Could you check a few things on this model? Use its own coordinates, in mm. Face numbers are marked on the shaded views. A direction names the side the tool comes from. Coordinates: 2 decimals unless noted, no trailing zeros. Order: outer loops, then holes, each group sorted by start corner. A loop starts at its lowest first (then second) coordinate and runs counter-clockwise, first axis right, second up. Notation, with made-up numbers: (-13, 49) - (13, 49) arc R22 cw to (13, 63) - close; hole circle Ø1 at (-26, 11.25). An arc over 180 degrees is marked (long way). One line per item, written item: value.
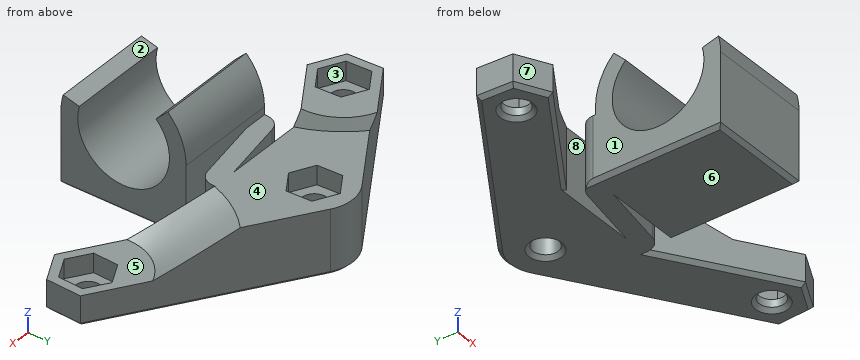
from build123d import *

# Parameters (mm, degrees)
BOSS_EXTRUDE1_DEPTH = 13.5
CUT_EXTRUDE1_DEPTH  = 19.454335534
SKETCH14_R          = 1.65
BOSS_EXTRUDE3_DEPTH = 8.5
CUT_EXTRUDE7_DEPTH  = 43.153930156
FILLET2_R           = 2
CUT_EXTRUDE9_DEPTH  = 4.5
CHAMFER2_SIZE       = 12
CHAMFER2_SIZE_2     = 6
CHAMFER3_SIZE       = 6
CHAMFER3_SIZE_2     = 12
CUT_EXTRUDE11_DEPTH = 2.5
CUT_EXTRUDE12_DEPTH = 2.5
CHAMFER4_SIZE       = 0.5
CHAMFER8_SIZE       = 0.5


with BuildPart() as part:
    # Sketch1 → Boss-Extrude1 (new body)
    with BuildSketch(Plane.ZY):
        with BuildLine():
            Line((-9.5, 8.25), (-9.5, -8.25))
            Line((-9.5, -8.25), (0, -8.25))
            ThreePointArc((0, -8.25), (8.25, 0), (0, 8.25))
            Line((0, 8.25), (-9.5, 8.25))
        make_face()
    extrude(amount=BOSS_EXTRUDE1_DEPTH)

    # Sketch7 → Cut-Extrude1 (cut, through all)
    with BuildSketch(Plane.ZY.offset(13.5)):
        with BuildLine():
            Line((13.481907846, 13.481907846), (4.277996026, 4.277996026))
            ThreePointArc((4.277996026, 4.277996026), (-5.843851249, 1.565855223), (1.565855223, -5.843851249))
            Line((1.565855223, -5.843851249), (4.934720763, -18.416628609))
            Line((4.934720763, -18.416628609), (13.481907846, 13.481907846))
        make_face()
    extrude(amount=-CUT_EXTRUDE1_DEPTH, mode=Mode.SUBTRACT)

    # Sketch14 → Boss-Extrude3 (add)
    with BuildSketch(Plane(origin=(0, 0, -9.5), x_dir=(-1, 0, 0), z_dir=(0, 0, -1))):
        with BuildLine():
            Line((4.039848555, 24.201794753), (-19.358847021, 9.109670469))
            Line((-19.358847021, 9.109670469), (-19.131451731, 4.496469334))
            Line((-19.131451731, 4.496469334), (-15.022604709, 2.386798865))
            Line((-15.022604709, 2.386798865), (0, 12.07635684))
            Line((0, 12.07635684), (0, 8.25))
            Line((0, 8.25), (13.5, 8.25))
            Line((13.5, 8.25), (13.5, 12.07635684))
            Line((13.5, 12.07635684), (28.522604709, 2.386798865))
            Line((28.522604709, 2.386798865), (32.631451731, 4.496469334))
            Line((32.631451731, 4.496469334), (32.858847021, 9.109670469))
            Line((32.858847021, 9.109670469), (9.460151445, 24.201794753))
            ThreePointArc((9.460151445, 24.201794753), (6.75, 25), (4.039848555, 24.201794753))
        make_face()
        with Locations((6.75, 20)):
            Circle(SKETCH14_R, mode=Mode.SUBTRACT)
        with Locations((-15.25, 7)):
            Circle(SKETCH14_R, mode=Mode.SUBTRACT)
        with Locations(Location((28.75, 7, 0), (0, 0, 180))):
            Circle(SKETCH14_R, mode=Mode.SUBTRACT)
    extrude(amount=-BOSS_EXTRUDE3_DEPTH)

    # Sketch15 → Cut-Extrude7 (cut, through all)
    with BuildSketch(Plane.XY.offset(-1)):
        Polygon((0, 8.25), (-10.401710887, 8.25), (0, 10.084102275), align=None)
        Polygon((-13.5, 10.242254565), (-13.5, 12.07635684), (-3.098289113, 12.07635684), align=None)
    extrude(amount=-CUT_EXTRUDE7_DEPTH, mode=Mode.SUBTRACT)

    # Fillet2
    fillet2_edges = [part.edges().sort_by_distance(p)[0] for p in [
        (0, 10.084102275, -5.25),
        (-13.5, 10.242254565, -5.25),
    ]]
    fillet(fillet2_edges, radius=FILLET2_R)

    # Sketch17 → Cut-Extrude9 (cut)
    with BuildSketch(Plane.XY.offset(-1)):
        with BuildLine():
            Line((19.131451731, 4.496469334), (19.358847021, 9.109670469))
            Line((19.358847021, 9.109670469), (17.418121156, 10.361435802))
            ThreePointArc((17.418121156, 10.361435802), (11.888564198, 9.168121156), (13.081878844, 3.638564198))
            Line((13.081878844, 3.638564198), (15.022604709, 2.386798865))
            Line((15.022604709, 2.386798865), (19.131451731, 4.496469334))
        make_face()
        with BuildLine():
            Line((-32.631451731, 4.496469334), (-28.522604709, 2.386798865))
            Line((-28.522604709, 2.386798865), (-26.581878844, 3.638564198))
            ThreePointArc((-26.581878844, 3.638564198), (-25.388564198, 9.168121156), (-30.918121156, 10.361435802))
            Line((-30.918121156, 10.361435802), (-32.858847021, 9.109670469))
            Line((-32.858847021, 9.109670469), (-32.631451731, 4.496469334))
        make_face()
    extrude(amount=-CUT_EXTRUDE9_DEPTH, mode=Mode.SUBTRACT)

    # Chamfer2
    # the kernel refuses this chamfer: 12, 6 mm, written as the material it takes off along each edge
    with BuildSketch(Plane(origin=(-28.75, 7, -1), x_dir=(-0.8386519680093931, -0.5446676753342096, 0), z_dir=(-0.5446676753342096, 0.8386519680093931, 0))) as chamfer2_piece_1_section:
        Polygon((4 + CHAMFER2_SIZE, 0), (4, -CHAMFER2_SIZE_2), (4, 0), align=None)
    chamfer2_piece_1 = revolve(axis=Axis((-28.75, 7, -1), (0, 0, 1)), revolution_arc=359.64, mode=Mode.PRIVATE)
    chamfer2_piece_1 = split(chamfer2_piece_1, bisect_by=Plane(origin=(-26.581878844, 3.638564198, -1), z_dir=(-0.5420302889814643, 0.8403589505840171, 0)), keep=Keep.TOP, mode=Mode.PRIVATE)
    chamfer2_piece_1 = split(chamfer2_piece_1, bisect_by=Plane(origin=(-28.75, 7, -5.5), z_dir=(0, 0, 1)), keep=Keep.TOP, mode=Mode.PRIVATE)
    add(chamfer2_piece_1, mode=Mode.SUBTRACT)

    # Chamfer3
    # the kernel refuses this chamfer: 12, 6 mm, written as the material it takes off along each edge
    with BuildSketch(Plane(origin=(15.25, 7, -1), x_dir=(0.8420576391550663, -0.5393875530085916, 0), z_dir=(-0.5393875530085916, -0.8420576391550663, 0))) as chamfer3_piece_1_section:
        Polygon((4, -CHAMFER3_SIZE), (4 + CHAMFER3_SIZE_2, 0), (4, 0), align=None)
    chamfer3_piece_1 = revolve(axis=Axis((15.25, 7, -1), (0, 0, 1)), revolution_arc=359.64, mode=Mode.PRIVATE)
    chamfer3_piece_1 = split(chamfer3_piece_1, bisect_by=Plane(origin=(15.25, 7, -5.5), z_dir=(0, 0, 1)), keep=Keep.TOP, mode=Mode.PRIVATE)
    chamfer3_piece_1 = split(chamfer3_piece_1, bisect_by=Plane(origin=(0, 7, -1), z_dir=(1, 0, 0)), keep=Keep.TOP, mode=Mode.PRIVATE)
    add(chamfer3_piece_1, mode=Mode.SUBTRACT)

    # Sketch19 → Cut-Extrude11 (cut)
    with BuildSketch(Plane.XY.offset(-5.5)):
        Polygon((-31.515534358, 5.2162344), (-28.587980855, 3.713094191), (-25.822446497, 5.496859791), (-25.984465642, 8.7837656), (-28.912019145, 10.286905809), (-31.677553503, 8.503140209), align=None)
        Polygon((18.015534358, 5.2162344), (18.177553503, 8.503140209), (15.412019145, 10.286905809), (12.484465642, 8.7837656), (12.322446497, 5.496859791), (15.087980855, 3.713094191), align=None)
    extrude(amount=-CUT_EXTRUDE11_DEPTH, mode=Mode.SUBTRACT)

    # Sketch20 → Cut-Extrude12 (cut)
    with BuildSketch(Plane.XY.offset(-1)):
        Polygon((-9.515534358, 18.2162344), (-6.587980855, 16.713094191), (-3.822446497, 18.496859791), (-3.984465642, 21.7837656), (-6.912019145, 23.286905809), (-9.677553503, 21.503140209), align=None)
    extrude(amount=-CUT_EXTRUDE12_DEPTH, mode=Mode.SUBTRACT)

    # Chamfer4
    chamfer4_edges = [part.edges().sort_by_distance(p)[0] for p in [
        (-5.1, 20, -9.5),
        (16.9, 7, -9.5),
        (-30.4, 7, -9.5),
    ]]
    chamfer(chamfer4_edges, length=CHAMFER4_SIZE)

    # Chamfer8
    # the kernel refuses this chamfer: 0.5 mm, written as the material it takes off along each edge
    with BuildSketch(Plane(origin=(-13.5, 10.749985843, -9.5), x_dir=(1, 0, 0), z_dir=(0, -1, 0))) as chamfer8_piece_1:
        Polygon((CHAMFER8_SIZE, 0), (0, CHAMFER8_SIZE), (0, 0), align=None)
    extrude(amount=20.285827337, mode=Mode.SUBTRACT)
    with BuildSketch(Plane(origin=(-12.419431591, 12.773321877, -9.5), x_dir=(-0.5420302889814643, 0.8403589505840171, 0), z_dir=(-0.8403589505840171, -0.5420302889814643, 0))) as chamfer8_piece_2_section:
        Polygon((CHAMFER8_SIZE, 0), (0, -CHAMFER8_SIZE), (0, 0), align=None)
    chamfer8_piece_2 = extrude(amount=20.448097226, mode=Mode.PRIVATE)
    chamfer8_piece_2 = split(chamfer8_piece_2, bisect_by=Plane(origin=(-12.419431591, 12.07635684, -9.5), z_dir=(0, -1, 0)), keep=Keep.TOP, mode=Mode.PRIVATE)
    add(chamfer8_piece_2, mode=Mode.SUBTRACT)
    with BuildSketch(Plane(origin=(-27.378731078, 1.799481691, -9.5), x_dir=(0.4567570550126589, 0.8895914751705769, 0), z_dir=(-0.8895914751705769, 0.4567570550126589, 0)), Plane(origin=(-32.568146508, 3.212187123, -9.5), x_dir=(0.9987873439941226, 0.04923252458656117, 0), z_dir=(-0.04923252458656117, 0.9987873439941226, 0)), Plane(origin=(19.422152244, 10.39395268, -9.5), x_dir=(-0.9987873439941226, 0.049232524586561265, 0), z_dir=(-0.049232524586561265, -0.9987873439941226, 0)), Plane(origin=(20.275325362, 5.083786508, -9.5), x_dir=(-0.4567570550126585, 0.8895914751705769, 0), z_dir=(-0.889591475170577, -0.45675705501265856, 0))) as chamfer8_piece_3:
        Polygon((CHAMFER8_SIZE, 0), (0, -CHAMFER8_SIZE), (0, 0), align=None)
    extrude(amount=7.190485141, mode=Mode.SUBTRACT)
    with BuildSketch(Plane(origin=(-33.93941543, 8.412705433, -9.5), x_dir=(0.5420302889814647, -0.8403589505840169, 0), z_dir=(0.8403589505840168, 0.5420302889814647, 0)), Plane(origin=(-4.039848555, 24.201794753, -9.5), x_dir=(-0.5420302889814645, -0.840358950584017, 0), z_dir=(0.8403589505840169, -0.5420302889814645, 0))) as chamfer8_piece_4:
        Polygon((CHAMFER8_SIZE, 0), (0, -CHAMFER8_SIZE), (0, 0), align=None)
    extrude(amount=29.12953324, mode=Mode.SUBTRACT)
    with BuildSketch(Plane(origin=(-6.75, 20, -9.5), x_dir=(-0.5420302889814639, 0.8403589505840172, 0), z_dir=(-0.8403589505840172, -0.5420302889814639, 0))) as chamfer8_piece_5:
        Polygon((5 - CHAMFER8_SIZE, 0), (5, -CHAMFER8_SIZE), (5, 0), align=None)
    revolve(axis=Axis((-6.75, 20, -9.5), (0, 0, -1)), revolution_arc=65.643913307, mode=Mode.SUBTRACT)
    with BuildSketch(Plane(origin=(16.103173118, 1.689833828, -9.5), x_dir=(0.5420302889814647, 0.8403589505840168, 0), z_dir=(-0.8403589505840168, 0.5420302889814647, 0))) as chamfer8_piece_6_section:
        Polygon((CHAMFER8_SIZE, 0), (0, -CHAMFER8_SIZE), (0, 0), align=None)
    chamfer8_piece_6 = extrude(amount=20.448097226, mode=Mode.PRIVATE)
    chamfer8_piece_6 = split(chamfer8_piece_6, bisect_by=Plane(origin=(0, 1.689833828, -9.5), z_dir=(1, 0, 0)), keep=Keep.TOP, mode=Mode.PRIVATE)
    add(chamfer8_piece_6, mode=Mode.SUBTRACT)
    with BuildSketch(Plane(origin=(0, -9.535841494, -9.5), x_dir=(-1, 0, 0), z_dir=(0, 1, 0))) as chamfer8_piece_7:
        Polygon((CHAMFER8_SIZE, 0), (0, CHAMFER8_SIZE), (0, 0), align=None)
    extrude(amount=19.071682988, mode=Mode.SUBTRACT)
    with BuildSketch(Plane(origin=(1.285841494, -8.25, -9.5), x_dir=(0, 1, 0), z_dir=(-1, 0, 0))) as chamfer8_piece_8:
        Polygon((CHAMFER8_SIZE, 0), (0, -CHAMFER8_SIZE), (0, 0), align=None)
    extrude(amount=16.071682988, mode=Mode.SUBTRACT)


solid = part.part
Item 1: I'm going to push flat-ended pins straight in: pin 1 Ø5 at (y, z) = (11, -0.5) entering from +X; pin 2 Ø3 at (x, y) = (-7, 19) entering from +Z; pin 3 Ø5 at (x, y) = (12.5, 11) entering from +Z; pin 4 Ø2 at (x, y) = (-28.75, 7) entering from -Z. Where does each tip first touch, or does it pass through?
Conclusion:
pin 1: x = 4.02
pin 2: z = -3.5
pin 3: z = -5.32
pin 4: through
Item 2: Thinking about a two-plate mould opening in X: for the marked faces 6, 7 and 8, which applies, pulls with the +X half, pulls with the -X half, needs draft (parallel to the pull), parting line crosses it, or undercut?
Conclusion:
face 6: needs draft
face 7: pulls with the -X half
face 8: undercut
Item 3: If I drill on probe 1 along Y at (x, z) = (-6.75, -6.6); probe 2 along Y at (x, z) = (-6.75, -5); probe 3 along Z at (x, y) = (-13.5, 17), over which ranges is the centre line in solid material (lowest first)?
Conclusion:
probe 1: -8.25 to 8.25, 8.89 to 11.43, 12.08 to 18.35, 21.65 to 25
probe 2: -8.25 to -3.41, 3.41 to 8.25, 8.89 to 11.43, 12.08 to 18.35, 21.65 to 25
probe 3: -9.5 to -1
Item 4: For the marked faces 1, 2, 3, 4 and 5, which set-ups out of +Z, -Z, +X, -X, +Y, -Y let a thin tool reach every point of the face, with its end or its side?
Conclusion:
face 1: +Z, -Z, -Y
face 2: +Z, +X, -X
face 3: +Z
face 4: +Z, +X, -X, +Y
face 5: +Z, +X, -Y
Item 5: I want a section at A-A on y = 0. Please give me the cut outline in (x, z), then the cut area to 3 significant figures.
Conclusion:
outline: (-13.5, -9) - (-13, -9.5) - (-0.5, -9.5) - (0, -9) - (0, -6.05) - (-13.5, -6.05) - close
area: 46.3 mm²
